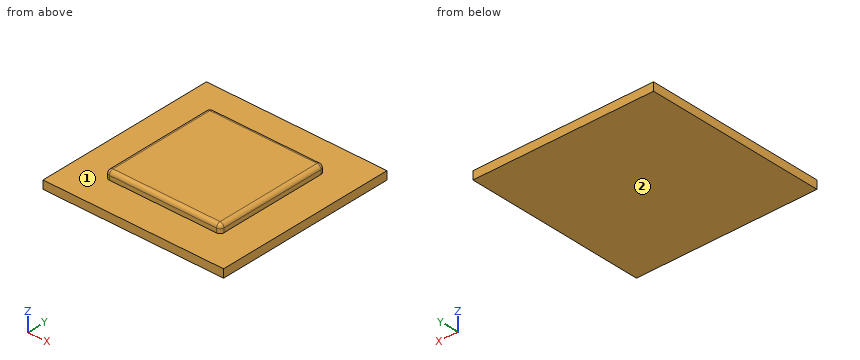
```python
from build123d import *

# Parameters (mm, degrees)
F0_W     = 88.9
F0_H     = 88.9
F1_DEPTH = 12.7
F0_W_2   = 139.7
F0_H_2   = 139.7
F2_DEPTH = 6.4
F3_R     = 3


with BuildPart() as f1:
    # F0 (on Top) → F1 (new body)
    with BuildSketch(Plane.XY):
        with Locations((-23.846633, 1.028963)):
            Rectangle(F0_W, F0_H)
    extrude(amount=F1_DEPTH)

    # F0 (on Top) → F2 (join)
    with BuildSketch(Plane.XY):
        with Locations((-23.846633, 1.028963)):
            Rectangle(F0_W_2, F0_H_2)
        with Locations((-23.846633, 1.028963)):
            Rectangle(F0_W, F0_H, mode=Mode.SUBTRACT)
    extrude(amount=F2_DEPTH)

    # F3
    f3_edges = [f1.edges().sort_by_distance(p)[0] for p in [
        (-68.296633, 1.028963, 12.7),
        (-23.846633, -43.421037, 12.7),
        (20.603367, 1.028963, 12.7),
        (-23.846633, 45.478963, 12.7),
        (20.603367, -43.421037, 9.55),
        (-68.296633, -43.421037, 9.55),
        (-68.296633, 45.478963, 9.55),
        (20.603367, 45.478963, 9.55),
    ]]
    fillet(f3_edges, radius=F3_R)


solid = f1.part
```
The listing builds one solid part. Answer for the finished solid, in the listing's coordinates (mm). Face numbers are marked on the shaded views. A direction names the side the tool comes from. Round coordinates to 2 decimals unless told otherwise and drop trailing zeros. Loops run counter-clockwise (first coordinate to the right, second up) from the corner with the lowest first, then second, coordinate; pieces in that order, holes last.
1) A cutting plane is placed at C-C on x = -6. Determine the outline of the cut face in (y, z), plus the area to 3 significant figures.
Outcome:
outline: (-68.82, 0) - (70.88, 0) - (70.88, 6.4) - (45.48, 6.4) - (45.48, 9.7) arc R3 ccw to (42.48, 12.7) - (-40.42, 12.7) arc R3 ccw to (-43.42, 9.7) - (-43.42, 6.4) - (-68.82, 6.4) - close
area: 1,450 mm2
2) For the marked faces 1 and 2, determine the directions among +Z, -Z, +X, -X, +Y, -Y from which every point of the face is accessible in a straight line to the end or side of a thin tool.
Outcome:
face 1: +Z
face 2: -Z, +X, -X, +Y, -Y
3) Given P1, Ø1.6, axis at x = -41, z = 8.5, coming from the -Y side; P2, Ø5, axis at y = 46.5, z = 9, coming from the -X side; P3, Ø2.5, axis at x = -8.5, z = 8.5, coming from the +Y side, each flat-ended and moving along its own axis, determine where each tip first touches the part or whether it passes through.
Outcome:
P1: stops at y = -43.42
P2: stops at x = -67.88
P3: stops at y = 45.48
4) A cutting plane is placed at B-B on y = -15. Determine the outline of the cut face in (x, z).
Outcome:
outline: (-93.7, 0) - (46, 0) - (46, 6.4) - (20.6, 6.4) - (20.6, 9.7) arc R3 ccw to (17.6, 12.7) - (-65.3, 12.7) arc R3 ccw to (-68.3, 9.7) - (-68.3, 6.4) - (-93.7, 6.4) - close
5) A cutting plane is placed at D-D on y = -52.5. Determine the outline of the cut face in (x, z).
Outcome:
outline: (-93.7, 0) - (46, 0) - (46, 6.4) - (-93.7, 6.4) - close
6) Consider line 1 (Z direction, x = -84.5, y = -52); line 2 (X direction, y = -15.5, z = 7.5); line 3 (Y direction, x = 12, z = 9.5). Determine where each line is inside the solid, lowest interval first.
Outcome:
line 1: z = 0 to 6.4
line 2: x = -68.3 to 20.6
line 3: y = -43.42 to 45.48
7) A cutting plane is placed at A-A on z = 8. Determine the outline of the cut face in (x, y), plus the area to 3 significant figures.
Outcome:
outline: (-68.3, -40.42) arc R3 ccw to (-65.3, -43.42) - (17.6, -43.42) arc R3 ccw to (20.6, -40.42) - (20.6, 42.48) arc R3 ccw to (17.6, 45.48) - (-65.3, 45.48) arc R3 ccw to (-68.3, 42.48) - close
area: 7,900 mm2
